Source: CAD feature listing. Evaluate the final solid. Frame: model axes, mm. Face numbers are marked on the shaded views. A direction names the side the tool comes from. Give positions to 0.01 mm unless a question says otherwise; leave off trailing zeros. Order: outer loops, then holes, each group sorted by start corner. A loop starts at its lowest first (then second) coordinate and runs counter-clockwise, first axis right, second up.
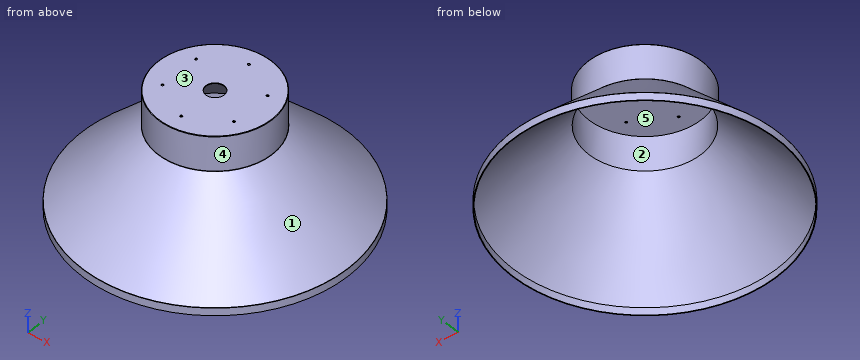
from build123d import *

# Parameters (mm, degrees)
F2_R     = 5
F3_DEPTH = 1.5
F4_R     = 20
F5_DEPTH = 254.001
F6_R     = 2.6
F7_DEPTH = 254.001


with BuildPart() as f1:
    # F0 (on Front) → F1 (revolve)
    with BuildSketch(Plane.XZ):
        with BuildLine():
            Line((288, 16), (288, 0))
            Line((288, 0), (289.5, 0))
            Line((289.5, 0), (289.5, 16.210244))
            ThreePointArc((289.5, 16.210244), (289.421822, 16.597858), (289.19951, 16.924867))
            Line((289.19951, 16.924867), (124.30049, 178.336596))
            ThreePointArc((124.30049, 178.336596), (124.078178, 178.663604), (124, 179.051219))
            Line((124, 179.051219), (124, 253))
            ThreePointArc((124, 253), (123.707107, 253.707107), (123, 254))
            Line((123, 254), (0, 254))
            Line((0, 254), (0, 252.5))
            Line((0, 252.5), (122.5, 252.5))
            Line((122.5, 252.5), (122.5, 178))
            Line((122.5, 178), (288, 16))
        make_face()
    revolve(axis=Axis((0, 0, 126.25), (0, 0, 1)))

    # F2 (on face) → F3 (cut, through all)
    with BuildSketch(Plane.XY.offset(254)):
        Circle(F2_R)
    extrude(amount=-F3_DEPTH, mode=Mode.SUBTRACT)

    # F4 (on face) → F5 (cut, through all)
    with BuildSketch(Plane.XY.offset(254)):
        Circle(F4_R)
    extrude(amount=-F5_DEPTH, mode=Mode.SUBTRACT)

    # F6 (on face) → F7 (cut, through all)
    with BuildSketch(Plane.XY.offset(254)):
        with Locations((0, 89.65)):
            Circle(F6_R)
        with Locations((-77.639177, 44.825)):
            Circle(F6_R)
        with Locations((-77.639177, -44.825)):
            Circle(F6_R)
        with Locations((0, -89.65)):
            Circle(F6_R)
        with Locations((77.639177, -44.825)):
            Circle(F6_R)
        with Locations((77.639177, 44.825)):
            Circle(F6_R)
    extrude(amount=-F7_DEPTH, mode=Mode.SUBTRACT)


solid = f1.part
1) Ray query, L1, parallel to Y at x = 0, z = 252.9; L2, parallel to Y at x = 0, z = 3; L3, parallel to Z at x = 21, y = -3.5. Return the intervals inside material, ascending.
Checks:
L1: y = -124 to -92.25, -87.05 to -20, 20 to 87.05, 92.25 to 124
L2: y = -289.5 to -288, 288 to 289.5
L3: z = 252.5 to 254
2) Section query C-C on z = 62. Output: boundary loops of the cut face in (x, y), and give its area (3 significant figures).
Checks:
outline: circle Ø486.3 at (0, 0); hole circle Ø482.01 at (0, 0)
area: 3,260 mm2
3) Reachability of the marked faces 1 and 2 from +Z, -Z, +X, -X, +Y, -Y: full face, straight path, thin tool, end or side. Return the list, or none.
Checks:
face 1: +Z
face 2: -Z
4) Pull-direction query (Y, two-part tool) for the marked faces 3, 4 and 5; classes: +Y half, -Y half, draft (parallel to the pull), parting line (faces both ways), or undercut.
Checks:
face 3: draft
face 4: parting line
face 5: undercut
5) Section query A-A on y = 0. Output: boundary loops of the cut face in (x, z).
Checks:
outline: (-289.5, 0) - (-288, 0) - (-288, 16) - (-122.5, 178) - (-122.5, 252.5) - (-20, 252.5) - (-20, 254) - (-123, 254) arc R1 ccw to (-124, 253) - (-124, 179.05) arc R1 cw to (-124.3, 178.34) - (-289.2, 16.92) arc R1 ccw to (-289.5, 16.21) - close; (20, 252.5) - (122.5, 252.5) - (122.5, 178) - (288, 16) - (288, 0) - (289.5, 0) - (289.5, 16.21) arc R1 ccw to (289.2, 16.92) - (124.3, 178.34) arc R1 cw to (124, 179.05) - (124, 253) arc R1 ccw to (123, 254) - (20, 254) - close
6) First-contact query: pin 1 Ø7 at (x, y) = (0, -89.65) entering from -Z; pin 2 Ø1.5 at (x, y) = (-154.5, 192.5) entering from +Z; pin 3 Ø12 at (x, y) = (175.5, 162) entering from +Z. Flat tips, straight axial feed; report the tip coordinate or a pass-through.
Checks:
pin 1: stops at z = 252.5
pin 2: stops at z = 59.13
pin 3: stops at z = 72.09
7) Section query B-B on z = 29. Output: boundary loops of the cut face in (x, y).
Checks:
outline: circle Ø553.73 at (0, 0); hole circle Ø549.44 at (0, 0)
